```python
from build123d import *
from build123d.topology import SkipClean

# Parameters (mm, degrees)
SKETCH3_R           = 7.5
BOSS_EXTRUDE1_DEPTH = 2


with BuildPart() as part:
    # Sketch3 → Boss-Extrude1 (new body)
    with BuildSketch(Plane(origin=(0, 0, 0), x_dir=(1, 0, 0), z_dir=(0, 1, 0))):
        with Locations(Location((0, 0, 0), (0, 0, 270))):
            Circle(SKETCH3_R)
    extrude(amount=-BOSS_EXTRUDE1_DEPTH)

    # Sketch4 → Revolve3 (revolve)
    with BuildSketch(Plane.XY):
        Polygon((0, -2), (0, -19), (-2.45, -19), (-2.45, -17), (-1.2, -17), (-1.2, -6), (-2.5, -6), (-2.5, -4.5), (-1.2, -4.5), (-1.2, -4), (-4, -2), align=None)
    revolve(axis=Axis((0, -2, 0), (0, -1, 0)))

    # Sketch5 → Revolve4 (revolve)
    with SkipClean():  # the faces are left unmerged after this step: merging them gives an invalid solid
        with BuildSketch(Plane(origin=(0, 0, 0), x_dir=(0, 0, -1), z_dir=(1, 0, 0))):
            with BuildLine():
                Line((-2, 0), (0, 0))
                Line((0, 0), (0, 16.1))
                ThreePointArc((0, 16.1), (-1.037371232, 16.24049725), (-2, 16.651866191))
                Line((-2, 16.651866191), (-2, 0))
            make_face()
            with BuildLine():
                ThreePointArc((-2, 16.651866191), (-1.037371232, 16.24049725), (0, 16.1))
                Line((0, 16.1), (0, 20))
                Line((0, 20), (0, 23.9))
                ThreePointArc((0, 23.9), (-3.75950275, 21.037371232), (-2, 16.651866191))
            make_face()
            with BuildLine():
                Line((0, 20), (0, 16.1))
                ThreePointArc((0, 16.1), (1.037371232, 16.24049725), (2, 16.651866191))
                ThreePointArc((2, 16.651866191), (3.391902121, 18.075162345), (3.9, 20))
                ThreePointArc((3.9, 20), (2.757716447, 22.757716447), (0, 23.9))
                Line((0, 23.9), (0, 20))
            make_face()
        revolve(axis=Axis((0, 0, 0), (0, 1, 0)))
    add(part.part.scale(1), mode=Mode.REPLACE)  # the faces are merged on a copy


solid = part.part
```
Read the model definition and answer for the solid it produces. Units are mm, in the model's axes. A direction names the side the tool comes from. Give positions to 0.01 mm unless a question says otherwise; leave off trailing zeros. Write each loop counter-clockwise with the first axis right and the second up, starting at its lowest first coordinate (ties: lowest second). Pieces come first, ordered by that corner, then holes. Notation, with made-up numbers: M 33,75 L 73,75 A25 ccw 73,105 Z; hole C 27.5,19.25 d9. An arc over 180 degrees is marked long. Put each result on its own line as item: value. Start each with the question number.
1. For a pull along Y with two mould halves and no side action, classify faces 1 (the conical face through (0.298, -3.875, 1.342)), 2 (the cylindrical face through (0.54, -5.24, 2.44)), 3 (the flat face through (-3, -2, 3)) as released by +Y, released by -Y, zero draft, split by the parting line, or undercut.
2. Each of these flat-tipped pins is pushed along its axis until it touches: pin 1 Ø3 at (x, y) = (-5.5, 3) entering from +Z (3 decimals); pin 2 Ø1.5 at (x, z) = (-0.5, 0.5) entering from +Y; pin 3 Ø6 at (x, z) = (3.5, -3) entering from +Y; pin 4 Ø2 at (x, y) = (2, 15.5) entering from -Z. Where does it stop, or does it pass through?
3. The part is cut by section C-C, the plane y = 12.5. Give the vertices of the cut face in (x, z), and give its area (3 significant figures).
4. The part is cut by section D-D, the plane x = 4.75. Give the vertices of the cut face in (y, z), and give its area (3 significant figures).
5. The part is cut by section A-A, the plane x = 0. Give the vertices of the cut face in (y, z), and give its area (3 significant figures).
6. Which of the six approach directions +Z, -Z, +X, -X, +Y, -Y give full straight-line access (tool end or side, diameter ignored) to faces 4 (the cylindrical face through (0.5, -18, 2.4)), 5 (the flat face through (0, -19, 0)), 6 (the cylindrical face through (-0.65, -11.42, -1.01))?
7. The part is cut by section B-B, the plane z = 0. Give the vertices of the cut face in (x, y).
8. Consider line 1 along Y through (x, z) = (4.25, -4); line 2 along Y through (x, z) = (2.25, 0.5); line 3 along X through (y, z) = (-16, 0.75). Determine where each line is inside the solid, lowest interval first.
Final values:
1. face 1: undercut
1. face 2: zero draft
1. face 3: released by -Y
2. pin 1: passes through
2. pin 2: stops at y = 23.9
2. pin 3: stops at y = 23.55
2. pin 4: stops at z = -1.73
3. outline: C 0,0 d4
3. area: 12.6 mm²
4. outline: M -2,-5.8 L 0,-5.8 L 0,5.8 L -2,5.8 Z
4. area: 23.2 mm²
5. outline: M -19,-2.45 L -17,-2.45 L -17,-1.2 L -6,-1.2 L -6,-2.5 L -4.5,-2.5 L -4.5,-1.2 L -4,-1.2 L -2,-4 L -2,-7.5 L 0,-7.5 L 0,-2 L 16.65,-2 A3.9 ccw long 16.65,2 L 0,2 L 0,7.5 L -2,7.5 L -2,4 L -4,1.2 L -4.5,1.2 L -4.5,2.5 L -6,2.5 L -6,1.2 L -17,1.2 L -17,2.45 L -19,2.45 Z
5. area: 198 mm²
6. face 4: -Y
6. face 5: +Z, -Z, +X, -X, -Y
6. face 6: none
7. outline: M -7.5,-2 L -4,-2 L -1.2,-4 L -1.2,-4.5 L -2.5,-4.5 L -2.5,-6 L -1.2,-6 L -1.2,-17 L -2.45,-17 L -2.45,-19 L 2.45,-19 L 2.45,-17 L 1.2,-17 L 1.2,-6 L 2.5,-6 L 2.5,-4.5 L 1.2,-4.5 L 1.2,-4 L 4,-2 L 7.5,-2 L 7.5,0 L 2,0 L 2,16.65 A3.9 ccw long -2,16.65 L -2,0 L -7.5,0 Z
8. line 1: y = -2 to 0
8. line 2: y = -19 to -17, -6 to -4.5, -3.21 to 0, 16.85 to 23.15
8. line 3: x = -0.94 to 0.94
